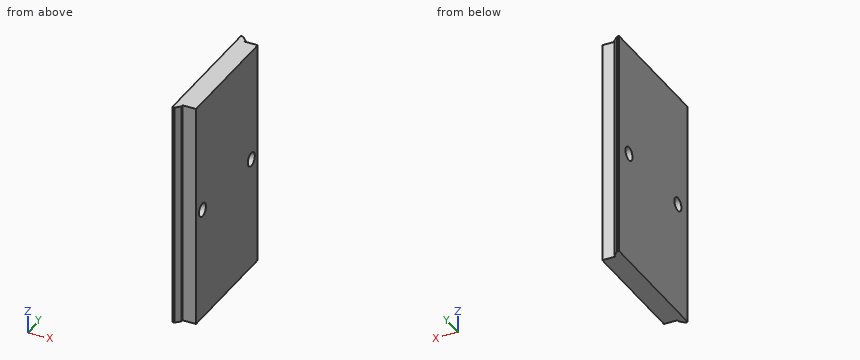
Autodesk Inventor part; units mm, degrees
ref_plane "YZ Plane" through (0, 0, 0) normal (1, 0, 0) x (0, 1, 0)
ref_plane "XZ Plane" through (0, 0, 0) normal (0, 1, 0) x (-1, 0, 0)
ref_plane "XY Plane" through (0, 0, 0) normal (0, 0, 1) x (1, 0, 0)
sketch "Sketch1" plane through (0, 0, 0) normal (0, 0, 1) x (1, 0, 0)
  line L0 (-19.2766, 29.5) -> (-19.2766, -29.4652)
  line L1 (-18.2766, -29.4652) -> (-19.2766, -29.4652)
  line L2 (-16.2766, -27.4652) -> (-18.2766, -29.4652)
  line L3 (-16.2766, -26.5) -> (-16.2766, -27.4652)
  line L4 (-16.2766, -26.5) -> (28.7234, -26.5) construction
  arc A0 (28.7234, -26.5) -> (30.7234, -24.5) centre (28.7234, -24.5) ccw
  line L5 (30.7234, -24.5) -> (30.7234, -19.5)
  line L6 (30.7234, -19.5) -> (27.7234, -22.5)
  line L7 (27.7234, -22.5) -> (-14.2766, -22.5) construction
  arc A1 (-16.2766, -20.5) -> (-14.2766, -22.5) centre (-14.2766, -20.5) ccw construction
  line L8 (-16.2766, -20.5) -> (-16.2766, 20.5) construction
  arc A2 (-14.2766, 22.5) -> (-16.2766, 20.5) centre (-14.2766, 20.5) ccw construction
  line L9 (-14.2766, 22.5) -> (27.7234, 22.5) construction
  line L10 (27.7234, 22.5) -> (30.7234, 19.5)
  line L11 (30.7234, 19.5) -> (30.7234, 24.5)
  arc A3 (30.7234, 24.5) -> (28.7234, 26.5) centre (28.7234, 24.5) ccw
  line L12 (28.7234, 26.5) -> (-16.2766, 26.5) construction
  line L13 (-16.2766, 26.5) -> (-16.2766, 27.5)
  line L14 (-16.2766, 27.5) -> (-18.2766, 29.5)
  line L15 (-18.2766, 29.5) -> (-19.2766, 29.5)
  line L16 (-16.2766, -26.5) -> (-10.2766, -26.5)
  line L17 (-10.2766, -26.5) -> (-10.2766, 26.5)
  line L18 (-10.2766, 26.5) -> (-16.2766, 26.5)
  line L19 (-10.2766, 26.5) -> (-16.2766, 26.5)
  line L20 (-19.2766, -29.4652) -> (-19.2766, 29.5)
  line L21 (-18.2766, 29.5) -> (-19.2766, 29.5)
  line L22 (-18.2766, 29.5) -> (-16.2766, 27.5)
  line L23 (-16.2766, 27.5) -> (-16.2766, 26.5)
  line L24 (-19.2766, -29.4652) -> (-18.2766, -29.4652)
  line L25 (-18.2766, -29.4652) -> (-16.2766, -27.4652)
  line L26 (-16.2766, -27.4652) -> (-16.2766, -26.5)
  point P0 (0, 0)
  dimension "d0" = 6
extrude "Extrusion1" add sketch "Sketch1" along normal blind 100
sketch "Sketch2" plane through (-10.2766, -26.5, 0) normal (1, 0, 0) x (0, 0, -1)
  line L0 (0, -2.9652) -> (0, -0.9652)
  line L1 (-100, 56) -> (-100, -2.9652)
  line L2 (0, -2.9652) -> (-100, -2.9652)
  line L3 (-100, 56) -> (-100, -2.9652)
  line L4 (0, 56) -> (0, -2.9652)
  line L5 (0, 56) -> (-100, 56)
  circle A0 centre (-50, 5.5174) radius 3
  circle A1 centre (-50, 47.5174) radius 3
  point P0 (0, 26.5)
  dimension "d5" = 6
  dimension "d6" = 6
extrude "Extrusion2" cut sketch "Sketch2" against normal blind 100 contours A0 | A1
scale "Scale1" factors (0.5, 0.5, 0.5) then translate (-9.6383, 0.0087, 25) bodies 1
properties part number "batteryholder9"
Part model, mm, in its own coordinate system. Coordinates: 2 decimals unless noted, no trailing zeros. Write each loop counter-clockwise with the first axis right and the second up, starting at its lowest first coordinate (ties: lowest second). Pieces come first, ordered by that corner, then holes.
Item 1: Slice it at A-A (z = 50). Write the cut outline in (x, y).
Item 2: Slice it at C-C (z = 57). Write the cut outline in (x, y).
Item 3: Probe line 1 (Y direction, x = -17.6, z = 50); line 2 (Y direction, x = -16.3, z = 64); line 3 (Z direction, x = -15.3, y = 9.25). List the from-to ranges inside material, lowest first.
Item 4: Pin check, flat tips, straight feed: pin 1 (1 mm diameter, centred on x = -15.5, z = 63, fed in from -Y); pin 2 (0.9 mm diameter, centred on x = -15.5, z = 44.5, fed in from +Y). Stop position of each tip, or through.
Item 5: Slice it at B-B (x = -16.7). Write the cut outline in (y, z), and give its area (3 significant figures).
Results found:
1. outline: (-19.28, -14.72) - (-18.78, -14.72) - (-17.78, -13.72) - (-17.78, -13.24) - (-14.78, -13.24) - (-14.78, -11.98) - (-19.28, -11.98) - close; (-19.28, -8.98) - (-14.78, -8.98) - (-14.78, 9.02) - (-19.28, 9.02) - close; (-19.28, 12.02) - (-14.78, 12.02) - (-14.78, 13.26) - (-17.78, 13.26) - (-17.78, 13.76) - (-18.78, 14.76) - (-19.28, 14.76) - close
2. outline: (-19.28, -14.72) - (-18.78, -14.72) - (-17.78, -13.72) - (-17.78, -13.24) - (-14.78, -13.24) - (-14.78, 13.26) - (-17.78, 13.26) - (-17.78, 13.76) - (-18.78, 14.76) - (-19.28, 14.76) - close
3. line 1: y = -13.24 to -11.98, -8.98 to 9.02, 12.02 to 13.26
3. line 2: y = -13.24 to 13.26
3. line 3: z = 25 to 49.2, 50.8 to 75
4. pin 1: stops at y = -13.24
4. pin 2: stops at y = 13.26
5. outline: (-13.24, 25) - (13.26, 25) - (13.26, 75) - (-13.24, 75) - close; hole circle Ø3 at (-10.48, 50); hole circle Ø3 at (10.52, 50)
5. area: 1,310 mm2
